from build123d import *

# Parameters (mm, degrees)
SKETCH2_R             = 201.031521777
BOSS_EXTRUDE7_DEPTH   = 4
BOSS_EXTRUDE7_2_DEPTH = 4
BOSS_EXTRUDE7_3_DEPTH = 4
BOSS_EXTRUDE10_DEPTH  = 6
BOSS_EXTRUDE11_DEPTH  = 8


with BuildPart() as part:
    # Sketch2 → Boss-Extrude7 (new body)
    with BuildSketch(Plane(origin=(0, 0, 0), x_dir=(1, 0, 0), z_dir=(0, 1, 0))):
        with Locations(Location((28.728301923, -36.999075156, 0), (0, 0, 270))):
            Circle(SKETCH2_R)
        Polygon((152.283015919, 111.685620156), (122.465283041, 72.187959679), (131.33927946, 61.588463956), (159.93326792, 73.282274115), (143.417774586, 47.455802993), (152.283015919, 36.866764734), (196.33706913, 58.705656004), (188.932474766, 67.550032606), (161.511800701, 55.272594698), (178.795417003, 80.987097248), (170.710153416, 90.644495422), (141.369313955, 77.507315286), (159.93326792, 102.547819155), align=None, mode=Mode.SUBTRACT)
        Polygon((8.355015654, 139.342235762), (8.355015654, 102.547819155), (-2.065397597, 102.547819155), (-2.065397597, 155.293154737), (13.798357886, 155.293154737), (27.918843536, 118.248670779), (42.300819661, 155.293154737), (57.990248161, 155.293154737), (57.990248161, 102.547819155), (47.617792653, 102.547819155), (47.617792653, 139.342235762), (33.550995269, 103.109575833), (22.166053086, 103.109575833), align=None, mode=Mode.SUBTRACT)
        with BuildLine():
            ThreePointArc((26.21202475, 88.771917484), (-60.995615689, 52.670789611), (-97.133377287, -34.521676642))
            Line((-97.133377287, -34.521676642), (26.186120795, -34.547580598))
            Line((26.186120795, -34.547580598), (26.21202475, 88.771917484))
        make_face(mode=Mode.SUBTRACT)
        with BuildLine():
            ThreePointArc((-97.133377287, -39.0255328), (-60.428579099, -125.690271204), (26.186120795, -162.512993196))
            Line((26.186120795, -162.512993196), (26.186120795, -39.0255328))
            Line((26.186120795, -39.0255328), (-97.133377287, -39.0255328))
        make_face(mode=Mode.SUBTRACT)
        with BuildLine():
            ThreePointArc((30.394002326, -162.512993196), (117.2962644, -125.8779667), (154.049264899, -39.0255328))
            Line((154.049264899, -39.0255328), (30.778576004, -39.0255328))
            Line((30.778576004, -39.0255328), (30.394002326, -162.512993196))
        make_face(mode=Mode.SUBTRACT)
        with BuildLine():
            ThreePointArc((154.049264899, -34.521676642), (117.203738276, 52.031920201), (30.605293957, 88.771917484))
            Line((30.605293957, 88.771917484), (30.605293957, -34.521676642))
            Line((30.605293957, -34.521676642), (154.049264899, -34.521676642))
        make_face(mode=Mode.SUBTRACT)
        with BuildLine():
            ThreePointArc((-106.417778138, 102.547819155), (-90.003173195, 105.01895685), (-83.698244067, 89.663383086))
            ThreePointArc((-83.698244067, 89.663383086), (-66.285464204, 87.446031309), (-65.417157073, 69.914129125))
            Line((-65.417157073, 69.914129125), (-94.990225375, 34.841498226))
            Line((-94.990225375, 34.841498226), (-135.009946729, 68.585928646))
            Line((-135.009946729, 68.585928646), (-106.417778138, 102.547819155))
        make_face(mode=Mode.SUBTRACT)
    extrude(amount=BOSS_EXTRUDE7_DEPTH)



with BuildPart() as body_2:
    # Sketch2 → Boss-Extrude7 2 (new body)
    with BuildSketch(Plane(origin=(0, 0, 0), x_dir=(1, 0, 0), z_dir=(0, 1, 0))):
        with BuildLine():
            ThreePointArc((-86.720953962, 78.679511972), (-77.810994424, 79.342936952), (-76.304147471, 70.536296052))
            Line((-76.304147471, 70.536296052), (-92.743706606, 50.992764213))
            Line((-92.743706606, 50.992764213), (-102.73694564, 59.398841753))
            Line((-102.73694564, 59.398841753), (-86.720953962, 78.679511972))
        make_face()
    extrude(amount=BOSS_EXTRUDE7_2_DEPTH)


with BuildPart() as body_3:
    # Sketch2 → Boss-Extrude7 3 (new body)
    with BuildSketch(Plane(origin=(0, 0, 0), x_dir=(1, 0, 0), z_dir=(0, 1, 0))):
        with BuildLine():
            ThreePointArc((-105.724699903, 89.663383086), (-96.957903767, 92.46322763), (-94.158059223, 83.696431494))
            Line((-94.158059223, 83.696431494), (-109.765335501, 65.257065635))
            Line((-109.765335501, 65.257065635), (-119.246794828, 73.282274115))
            Line((-119.246794828, 73.282274115), (-105.724699903, 89.663383086))
        make_face()
    extrude(amount=BOSS_EXTRUDE7_3_DEPTH)


with BuildPart() as part_1:
    add(part.part)

    add(body_2.part)  # Boss-Extrude10 merges body 2

    add(body_3.part)  # Boss-Extrude10 merges body 3
    # Sketch2_12 → Boss-Extrude10 (add)
    # profile 1 of 5: a face of its own
    with BuildSketch(Plane(origin=(0, 0, 0), x_dir=(1, 0, 0), z_dir=(0, 1, 0))):
        with BuildLine():
            ThreePointArc((-83.698244067, 89.663383086), (-66.285464204, 87.446031309), (-65.417157073, 69.914129125))
            Line((-65.417157073, 69.914129125), (-94.990225375, 34.841498226))
            Line((-94.990225375, 34.841498226), (-135.009946729, 68.585928646))
            Line((-135.009946729, 68.585928646), (-106.417778138, 102.547819155))
            ThreePointArc((-106.417778138, 102.547819155), (-90.003173195, 105.01895685), (-83.698244067, 89.663383086))
        make_face()
        with BuildLine():
            Line((-119.246794828, 73.282274115), (-105.724699903, 89.663383086))
            ThreePointArc((-105.724699903, 89.663383086), (-96.957903767, 92.46322763), (-94.158059223, 83.696431494))
            Line((-94.158059223, 83.696431494), (-109.765335501, 65.257065635))
            Line((-109.765335501, 65.257065635), (-119.246794828, 73.282274115))
        make_face(mode=Mode.SUBTRACT)
        with BuildLine():
            Line((-102.73694564, 59.398841753), (-86.720953962, 78.679511972))
            ThreePointArc((-86.720953962, 78.679511972), (-77.810994424, 79.342936952), (-76.304147471, 70.536296052))
            Line((-76.304147471, 70.536296052), (-92.743706606, 50.992764213))
            Line((-92.743706606, 50.992764213), (-102.73694564, 59.398841753))
        make_face(mode=Mode.SUBTRACT)
    # profile 2 of 5: a face of its own
    with BuildSketch(Plane(origin=(0, 0, 0), x_dir=(1, 0, 0), z_dir=(0, 1, 0))):
        Polygon((8.355015654, 102.547819155), (-2.065397597, 102.547819155), (-2.065397597, 155.293154737), (13.798357886, 155.293154737), (27.918843536, 118.248670779), (42.300819661, 155.293154737), (57.990248161, 155.293154737), (57.990248161, 102.547819155), (47.617792653, 102.547819155), (47.617792653, 139.342235762), (33.550995269, 103.109575833), (22.166053086, 103.109575833), (8.355015654, 139.342235762), align=None)
    # profile 3 of 5: a face of its own
    with BuildSketch(Plane(origin=(0, 0, 0), x_dir=(1, 0, 0), z_dir=(0, 1, 0))):
        Polygon((159.93326792, 102.547819155), (152.283015919, 111.685620156), (122.465283041, 72.187959679), (131.33927946, 61.588463956), (159.93326792, 73.282274115), (143.417774586, 47.455802993), (152.283015919, 36.866764734), (196.33706913, 58.705656004), (188.932474766, 67.550032606), (161.511800701, 55.272594698), (178.795417003, 80.987097248), (170.710153416, 90.644495422), (141.369313955, 77.507315286), align=None)
    # profile 4 of 5: a face of its own
    with BuildSketch(Plane(origin=(0, 0, 0), x_dir=(1, 0, 0), z_dir=(0, 1, 0))):
        with BuildLine():
            Line((154.049264899, -34.521676642), (30.605293957, -34.521676642))
            Line((30.605293957, -34.521676642), (30.605293957, 88.771917484))
            ThreePointArc((30.605293957, 88.771917484), (117.203738276, 52.031920201), (154.049264899, -34.521676642))
        make_face()
    # profile 5 of 5: a face of its own
    with BuildSketch(Plane(origin=(0, 0, 0), x_dir=(1, 0, 0), z_dir=(0, 1, 0))):
        with BuildLine():
            Line((26.186120795, -39.0255328), (-97.133377287, -39.0255328))
            ThreePointArc((-97.133377287, -39.0255328), (-60.428579099, -125.690271204), (26.186120795, -162.512993196))
            Line((26.186120795, -162.512993196), (26.186120795, -39.0255328))
        make_face()
    extrude(amount=BOSS_EXTRUDE10_DEPTH)

    # Sketch2_13 → Boss-Extrude11 (add)
    with BuildSketch(Plane(origin=(0, 0, 0), x_dir=(1, 0, 0), z_dir=(0, 1, 0))):
        with BuildLine():
            Line((26.186120795, -34.547580598), (26.21202475, 88.771917484))
            ThreePointArc((26.21202475, 88.771917484), (-60.995615689, 52.670789611), (-97.133377287, -34.521676642))
            Line((-97.133377287, -34.521676642), (26.186120795, -34.547580598))
        make_face()
        with BuildLine():
            Line((30.394002326, -162.512993196), (30.778576004, -39.0255328))
            Line((30.778576004, -39.0255328), (154.049264899, -39.0255328))
            ThreePointArc((154.049264899, -39.0255328), (117.2962644, -125.8779667), (30.394002326, -162.512993196))
        make_face()
    extrude(amount=BOSS_EXTRUDE11_DEPTH)


solid = part_1.part
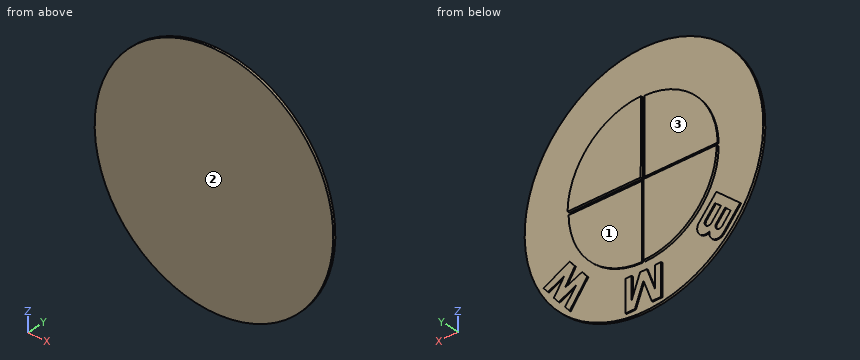
Verification items for the finished model (mm, model axes). Face numbers are marked on the shaded views. A direction names the side the tool comes from. Give positions to 0.01 mm unless a question says otherwise; leave off trailing zeros. Write each loop counter-clockwise with the first axis right and the second up, starting at its lowest first coordinate (ties: lowest second). Pieces come first, ordered by that corner, then holes. Notation, with made-up numbers: M 81,43.25 L 95,43.25 A35 cw 95,82.25 Z; hole C -21,38.25 d1. An arc over 180 degrees is marked long. Put each result on its own line as item: value. Start each with the question number.
1. Section check A-A (x = 76). Record the cut outline in (y, z).
2. Section check B-B (z = 46). Record the cut outline in (x, y).
3. Scan lines: line 1 along X through (y, z) = (4.75, -38); line 2 along Y through (x, z) = (90, -84); line 3 along X through (y, z) = (5.5, 116). Record each from-to range of solid material in increasing order. Write a range as [from, to].
4. Go/stop test with flat-tipped pins: pin 1 Ø1.6 at (y, z) = (5.5, -117.5) entering from +X; pin 2 Ø1.6 at (x, y) = (54, 5.5) entering from -Z; pin 3 Ø2 at (y, z) = (4.5, 80.5) entering from +X. Record where each tip stops, or that it passes through.
5. Section check D-D (z = 187). Record the cut outline in (x, y), and give its area (3 significant figures).
6. Set-up check for the marked faces 1, 2 and 3: record each of +Z, -Z, +X, -X, +Y, -Y from which the full face is reachable in a straight line by a thin tool's end or side.
7. Section check C-C (y = 1.25). Record the cut outline in (x, z).
Answer list:
1. outline: M 0,-158.4 L 4,-158.4 L 4,-79.42 L 6,-79.42 L 6,34.52 L 4,34.52 L 4,39.03 L 8,39.03 L 8,153.27 L 4,153.27 L 4,232.39 L 0,232.39 Z
2. outline: M -172.1,0 L 229.56,0 L 229.56,4 L 153.75,4 L 153.75,8 L 30.76,8 L 30.76,4 L 26.19,4 L 26.19,6 L -96.82,6 L -96.82,4 L -172.1,4 Z
3. line 1: [-98.74, -92.33], [-73.54, 26.2], [30.61, 129.32], [151.33, 154.57]
3. line 2: [0, 4]
3. line 3: [-69.15, 26.19], [30.54, 126.19]
4. pin 1: x = 57.99
4. pin 2: z = -155.29
4. pin 3: x = 225.19
5. outline: M -105.11,0 L 162.57,0 L 162.57,4 L -105.11,4 Z
5. area: 1,070 mm2
6. face 1: -Z, +X, +Y
6. face 2: +Z, -Z, +X, -X, -Y
6. face 3: +Z, -X, +Y
7. outline: C 28.73,37 d402.06
